Build history of the part. All positions in model axes, mm. Face numbers are marked on the shaded views. A direction names the side the tool comes from. Give positions to 0.01 mm unless a question says otherwise; leave off trailing zeros. Order: outer loops, then holes, each group sorted by start corner. A loop starts at its lowest first (then second) coordinate and runs counter-clockwise, first axis right, second up. Notation, with made-up numbers: (62.25, -7) - (105.25, -7) arc R21 cw to (105.25, -1) - close; hole circle Ø8 at (47, 65.25). An arc over 180 degrees is marked (long way). Write each question's results on one line, items separated by ' | '. Start each with the question number.
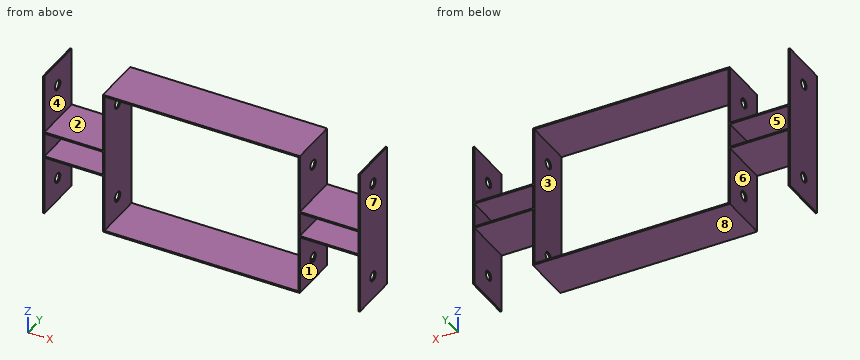
from build123d import *

# Parameters (mm, degrees)
SKETCH1_W               = 118.7
SKETCH1_H               = 49
SKETCH1_W_2             = 394
SKETCH1_H_2             = 289
BOSS_EXTRUDE1_DEPTH     = 100
CUT_EXTRUDE1_DEPTH      = 668.622505612
CUT_EXTRUDE1_DEPTH_BACK = 668.622505612
SKETCH3_R               = 10


with BuildPart() as part:
    # Sketch1 → Boss-Extrude1 (new body)
    with BuildSketch(Plane(origin=(0, 0, 0), x_dir=(1, 0, 0), z_dir=(0, 1, 0))):
        Polygon((200, 147.5), (-200, 147.5), (-200, 27.5), (-318.7, 27.5), (-318.7, 147.5), (-321.7, 147.5), (-321.7, -147.5), (-318.7, -147.5), (-318.7, -27.5), (-200, -27.5), (-200, -147.5), (200, -147.5), (200, -27.5), (318.7, -27.5), (318.7, -147.5), (321.7, -147.5), (321.7, 147.5), (318.7, 147.5), (318.7, 27.5), (200, 27.5), align=None)
        with Locations((259.35, 0)):
            Rectangle(SKETCH1_W, SKETCH1_H, mode=Mode.SUBTRACT)
        with Locations((-259.35, 0)):
            Rectangle(SKETCH1_W, SKETCH1_H, mode=Mode.SUBTRACT)
        Rectangle(SKETCH1_W_2, SKETCH1_H_2, mode=Mode.SUBTRACT)
    extrude(amount=BOSS_EXTRUDE1_DEPTH)

    # Sketch3 → Cut-Extrude1 (cut, two sides: drawn at the far end of the back side and taken through both)
    with BuildSketch(Plane(origin=(321.7, 0, 0), x_dir=(0, 0, -1), z_dir=(1, 0, 0)).offset(-CUT_EXTRUDE1_DEPTH_BACK)):
        with Locations(Location((-100, 48.5, 0), (0, 0, 180))):
            Circle(SKETCH3_R)
        with Locations(Location((100, 48.5, 0), (0, 0, 180))):
            Circle(SKETCH3_R)
    extrude(amount=CUT_EXTRUDE1_DEPTH + CUT_EXTRUDE1_DEPTH_BACK, mode=Mode.SUBTRACT)


solid = part.part
Item 1: Cut at B-B, the plane x = 276. List the corners of the cut face in (y, z).
Item 2: Cut at C-C, the plane z = -100. Count the separate pieces of the cut face and the enclosed holes in it, then the cut area to 3 significant figures.
Item 3: Flat gauge pins, fed straight in: pin 1 Ø23 at (y, z) = (48.5, -100) entering from +X; pin 2 Ø6 at (x, y) = (244, 64.5) entering from -Z. Where does each tip first touch, or does it go through?
Item 4: Cut at A-A, the plane z = 120. List the corners of the cut face in (x, y), then the cut area to 3 significant figures.
Item 5: Probe line 1 along X through (y, z) = (41, 59.5); line 2 along Z through (x, y) = (319, 48); line 3 along Z through (x, y) = (-85, 57). List the from-to ranges inside material, lowest first. Write a range as from..to.
Item 6: Two-plate mould, pull along Z, no slides. Class the marked faces 1, 2 and 3: +Z half, -Z half, draft (parallel to the pull), parting line (faces both ways), or undercut.
Item 7: Which spindle directions (+Z, -Z, +X, -X, +Y, -Y) get a long thin tool onto all of the face, cutting with end or side? Do the marked faces 4, 5, 6, 7 and 8. Say none if no direction does.
Values found:
1) outline: (0, -27.5) - (100, -27.5) - (100, -24.5) - (0, -24.5) - close; (0, 24.5) - (100, 24.5) - (100, 27.5) - (0, 27.5) - close
2) separate pieces: 8 | enclosed holes: 0 | area: 960 mm2
3) pin 1: stops at x = 321.7 | pin 2: stops at z = -27.5
4) outline: (-321.7, 0) - (-318.7, 0) - (-318.7, 100) - (-321.7, 100) - close; (-200, 0) - (-197, 0) - (-197, 100) - (-200, 100) - close; (197, 0) - (200, 0) - (200, 100) - (197, 100) - close; (318.7, 0) - (321.7, 0) - (321.7, 100) - (318.7, 100) - close | area: 1,200 mm2
5) line 1: x = -321.7..-318.7, -200..-197, 197..200, 318.7..321.7 | line 2: z = -147.5..-109.99, -90.01..90.01, 109.99..147.5 | line 3: z = -147.5..-144.5, 144.5..147.5
6) face 1: draft | face 2: +Z half | face 3: undercut
7) face 4: +Z, +Y, -Y | face 5: +Y, -Y | face 6: -Z, +Y, -Y | face 7: +Z, -Z, +X, +Y, -Y | face 8: -Z, +X, -X, +Y, -Y
